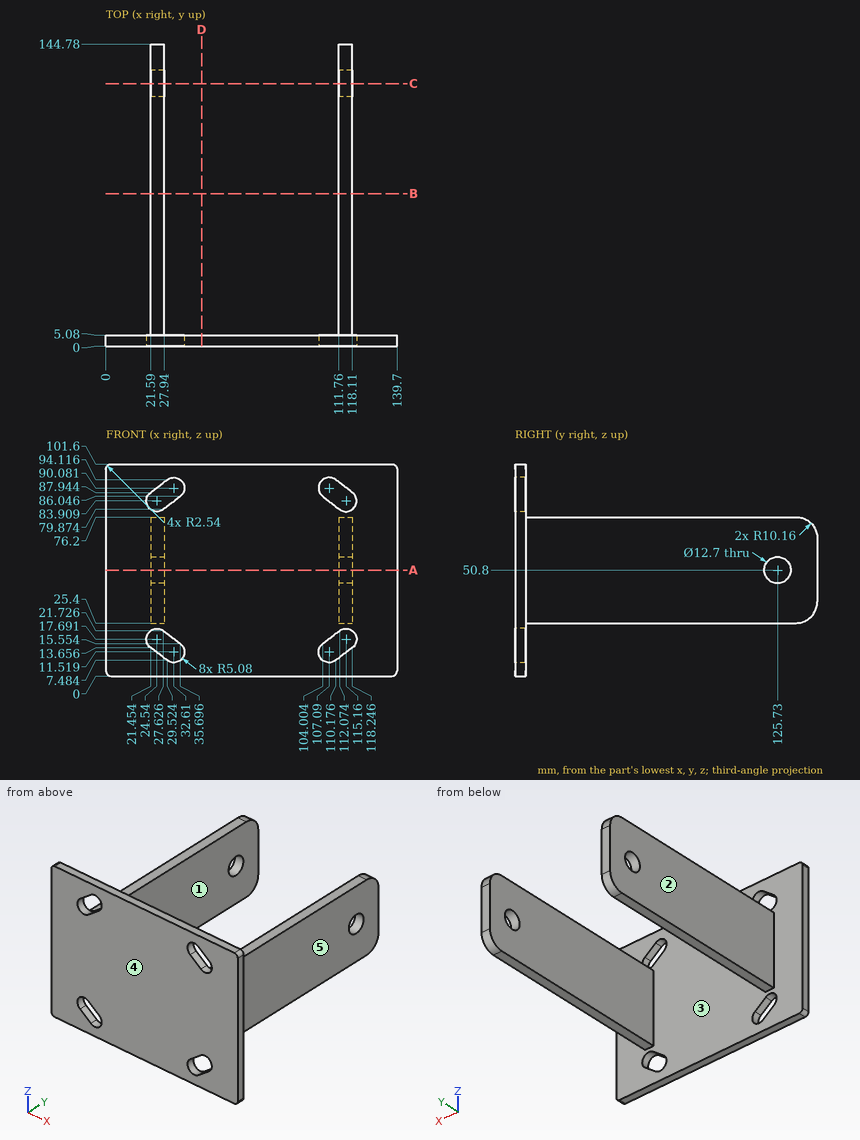
For this review, use the dimensioned drawing (mm, ordinates from the lowest corner) and the shaded views. A direction names the side the tool comes from. Give positions to 0.01 mm unless a question says otherwise; leave off trailing zeros. Write each loop counter-clockwise with the first axis right and the second up, starting at its lowest first coordinate (ties: lowest second). Pieces come first, ordered by that corner, then holes. Notation, with made-up numbers: M 1,2.5 L 22,2.5 A24 cw 22,35.5 Z; hole C 72.25,-33 d2. An arc over 180 degrees is marked long. Answer as a JSON object with one key per item and string values. Group by question number.
Item 1: For probe 1 along Y at (x, z) = (113.75, 50.8); probe 2 along X at (y, z) = (102.5, 69.5); probe 3 along Y at (x, z) = (35.5, 66), list the stretches that pass through material, from the lowest coordinate up. Write a range as [from, to].
Item 2: Consider section D-D on x = 46. Write out the cut boundary in (y, z), plus the area to 3 significant figures.
Item 3: Consider section A-A on z = 50.8. Write out the cut boundary in (x, y), plus the area to 3 significant figures.
Item 4: Consider section B-B on y = 73. Write out the cut boundary in (x, z), plus the area to 3 significant figures.
Item 5: Draft analysis for pull direction X (two halves, no side actions). For the marked faces 3, 4 and 5, state which applies: +X half, -X half, draft (parallel to the pull), parting line (faces both ways), or undercut.
Item 6: Consider section C-C on y = 125.73. Write out the cut boundary in (x, z).
Item 7: Tool access review of the marked faces 1 and 2: name each direction out of +Z, -Z, +X, -X, +Y, -Y from which nothing blocks a thin tool from reaching the whole face with its end or side.
Item 8: For pin 1 Ø2 at (x, y) = (117.5, 100) entering from -Z; pin 2 Ø14.5 at (y, z) = (125.73, 50.8) entering from +X; pin 3 Ø10 at (y, z) = (125.73, 50.8) entering from +X; pin 4 Ø1 at (x, z) = (57.5, 56.5) entering from -Y, all flat-tipped, find the tip position at first contact; note any pin that passes through.
Check result:
{
 "1": {"probe 1": "y = [0, 119.38], [132.08, 144.78]", "probe 2": "x = [21.59, 27.94], [111.76, 118.11]", "probe 3": "y = [0, 5.08]"},
 "2": {"outline": "M 0,0 L 5.08,0 L 5.08,101.6 L 0,101.6 Z", "area": "516 mm^2"},
 "3": {"outline": "M 0,0 L 139.7,0 L 139.7,5.08 L 118.11,5.08 L 118.11,119.38 L 111.76,119.38 L 111.76,5.08 L 27.94,5.08 L 27.94,119.38 L 21.59,119.38 L 21.59,5.08 L 0,5.08 Z; M 21.59,132.08 L 27.94,132.08 L 27.94,144.78 L 21.59,144.78 Z; M 111.76,132.08 L 118.11,132.08 L 118.11,144.78 L 111.76,144.78 Z", "area": "2,320 mm^2"},
 "4": {"outline": "M 21.59,25.4 L 27.94,25.4 L 27.94,76.2 L 21.59,76.2 Z; M 111.76,25.4 L 118.11,25.4 L 118.11,76.2 L 111.76,76.2 Z", "area": "645 mm^2"},
 "5": {"face 3": "undercut", "face 4": "draft", "face 5": "+X half"},
 "6": {"outline": "M 21.59,25.4 L 27.94,25.4 L 27.94,44.45 L 21.59,44.45 Z; M 21.59,57.15 L 27.94,57.15 L 27.94,76.2 L 21.59,76.2 Z; M 111.76,25.4 L 118.11,25.4 L 118.11,44.45 L 111.76,44.45 Z; M 111.76,57.15 L 118.11,57.15 L 118.11,76.2 L 111.76,76.2 Z"},
 "7": {"face 1": "+Z, -Z, +Y", "face 2": "+Z, -Z, -X, +Y"},
 "8": {"pin 1": "stops at z = 25.4", "pin 2": "stops at x = 118.11", "pin 3": "passes through", "pin 4": "stops at y = 0"}
}
